from build123d import *

# Parameters (mm, degrees)
F0_W          = 210
F0_H          = 225
F1_DEPTH      = 25
F3_DEPTH      = 95
F4_R          = 40
F5_DEPTH      = 10
F5_DEPTH_BACK = 127
F6_R          = 37.5
F7_DEPTH      = 10
F7_DEPTH_BACK = 127


with BuildPart() as f1:
    # F0 (on Top) → F1 (new body)
    with BuildSketch(Plane.XY):
        Rectangle(F0_W, F0_H)
    extrude(amount=F1_DEPTH)

    # F2 (on face) → F3 (join)
    with BuildSketch(Plane.XY.offset(25)):
        with BuildLine():
            Line((-71, -32.5), (-71, -112.5))
            Line((-71, -112.5), (-56, -112.5))
            Line((-56, -112.5), (-56, -46.4818166789))
            ThreePointArc((-56, -46.4818166789), (7.4888527117, -14.9888527117), (38.9818166789, 48.5))
            Line((38.9818166789, 48.5), (105, 48.5))
            Line((105, 48.5), (105, 63.5))
            Line((105, 63.5), (25, 63.5))
            ThreePointArc((25, 63.5), (-3.1177490061, -4.3822509939), (-71, -32.5))
        make_face()
    extrude(amount=F3_DEPTH)

    # F4 (on face) → F5 (join, two sides)
    with BuildSketch(Plane.YZ.offset(105)) as f5_sk:
        with Locations((56, 120)):
            Circle(F4_R)
    extrude(amount=F5_DEPTH)
    extrude(f5_sk.sketch, amount=-F5_DEPTH_BACK)

    # F6 (on face) → F7 (join, two sides)
    with BuildSketch(Plane.XZ.offset(112.5)) as f7_sk:
        with Locations((-63.5, 120)):
            Circle(F6_R)
        with BuildLine():
            ThreePointArc((-56, 83.2576538583), (-34.4526249034, 96.2829175487), (-26, 120))
            ThreePointArc((-26, 120), (-87.2170824513, 149.0473750966), (-71, 83.2576538583))
            Line((-71, 83.2576538583), (-71, 120))
            Line((-71, 120), (-56, 120))
            Line((-56, 120), (-56, 83.2576538583))
        make_face()
    extrude(amount=F7_DEPTH)
    extrude(f7_sk.sketch, amount=-F7_DEPTH_BACK)


solid = f1.part
The listing builds one solid part. Answer for the finished solid, in the listing's coordinates (mm). A direction names the side the tool comes from. Coordinates: 2 decimals unless noted, no trailing zeros. Loops run counter-clockwise (first coordinate to the right, second up) from the corner with the lowest first, then second, coordinate; pieces in that order, holes last.
1) A tool of negligible diameter and unlimited length cuts with its end or side. For faces 5 (the face through (-22, 55, 121)), 6 (the face through (41, -49, 25)), 7 (the face through (66, 63.5, 52)), 8 (the face through (-8, -112.5, 17)), 9 (the face through (-2.375, -3.632, 61.279)), from which of +Z, -Z, +X, -X, +Y, -Y can it reach the whole face along a straight path? Write none if from no direction.
2) Find the intervals of material crossed by L1, parallel to X at y = 76, z = 147.5; L2, parallel to X at y = -3.5, z = 16.5; L3, parallel to Y at x = 50.5, z = 57, in increasing order.
3) Find section C-C on z = 136. Write down the section's boundary in (x, y).
4) Determine the mould class of faces 1 (the face through (-1, -9, 120)), 2 (the face through (72, 48.5, 52)), 3 (the face through (-1, 2, 0)), 4 (the face through (-105, -2, 12)) for opening direction Z: pulls with the +Z half, pulls with the -Z half, needs draft (parallel to the pull), parting line crosses it, or undercut.
5) Find section B-B on x = 83.5. Write down the section's boundary in (y, z), then the cut area to 3 significant figures.
6) Flat-ended cylindrical pins translate along their axes: pin 1 Ø3 at (x, z) = (33.5, 56) entering from -Y; pin 2 Ø22.5 at (x, z) = (-55.5, 129) entering from +Y; pin 3 Ø16 at (x, y) = (-4.5, -3.5) entering from +Z; pin 4 Ø5 at (x, y) = (45.5, 9) entering from -Z. Find the tip coordinate at first contact, or state that the pin passes through.
7) Find section A-A on y = -57. Write down the section's boundary in (x, z).
8) Find section D-D on z = 88.5. Write down the section's boundary in (x, y), then the cut area to 3 significant figures.
Values:
1. face 5: +Z, -X, +Y
1. face 6: +X, -Y
1. face 7: +X, -X, +Y
1. face 8: -Z, +X, -X, -Y
1. face 9: none
2. L1: x = -22 to 115
2. L2: x = -105 to 105
2. L3: y = 48.5 to 63.5
3. outline: (-97.42, -122.5) - (-29.58, -122.5) - (-29.58, 14.5) - (-97.42, 14.5) - close; (-22, 19.34) - (115, 19.34) - (115, 92.66) - (-22, 92.66) - close
4. face 1: pulls with the +Z half
4. face 2: undercut
4. face 3: pulls with the -Z half
4. face 4: needs draft
5. outline: (-112.5, 0) - (112.5, 0) - (112.5, 25) - (63.5, 25) - (63.5, 80.71) arc R40 ccw (long way) to (48.5, 80.71) - (48.5, 25) - (-112.5, 25) - close
5. area: 11,500 mm2
6. pin 1: stops at y = 22.12
6. pin 2: stops at y = 14.5
6. pin 3: stops at z = 120
6. pin 4: stops at z = 0
7. outline: (-105, 0) - (105, 0) - (105, 25) - (-56, 25) - (-56, 83.26) arc R37.5 ccw (long way) to (-71, 83.26) - (-71, 25) - (-105, 25) - close
8. outline: (-83.85, -122.5) - (-43.15, -122.5) - (-43.15, -43.95) arc R111 ccw to (35.24, 31.35) - (115, 31.35) - (115, 80.65) - (-22, 80.65) - (-22, 31.35) - (19.46, 31.35) arc R96 cw to (-43.15, -28.37) - (-43.15, 14.5) - (-83.85, 14.5) - close
8. area: 13,900 mm2
